Input: part model. Units: mm. Frame: model coordinates. Face numbers are marked on the shaded views. Round coordinates to 2 decimals unless told otherwise and drop trailing zeros. Loops run counter-clockwise (first coordinate to the right, second up) from the corner with the lowest first, then second, coordinate; pieces in that order, holes last.
(1) Line query: line 1 (Y direction, x = 232.1, z = 2.05); line 2 (X direction, y = 23, z = 2.8); line 3 (Z direction, x = 208.5, y = 32). Output: solid intervals per line, ascending.
(2) First-contact query: pin 1 Ø8.5 at (x, y) = (232.1, 71.1) entering from +Z; pin 2 Ø4.5 at (x, y) = (94.1, 23.7) entering from +Z. Flat tips, straight axial feed; report the tip coordinate or a pass-through.
(3) Cut plane C-C, the plane y = 48.5. Output: boundary loops of the cut face in (x, z).
(4) Draft query along Y for the marked faces 1 and 2. Return one class per face: released by +Y, released by -Y, zero draft, split by the parting line, or undercut.
(5) Cut plane A-A, the plane y = 23.7. Output: boundary loops of the cut face in (x, z).
(6) Cut plane B-B, the plane x = 13.6. Output: boundary loops of the cut face in (y, z) (3 decimals).
(7) Cut plane D-D, the plane x = 120. Output: boundary loops of the cut face in (y, z), and give its area (3 significant figures).
from build123d import *

# Parameters (mm, degrees)
SKETCH1_W                = 257.2
SKETCH1_H                = 94.8
BOSS_EXTRUDE1_DEPTH      = 3
SKETCH2_R                = 2.995
BOSS_EXTRUDE2_DEPTH      = 1.4
LPATTERN1_COUNT          = 2
LPATTERN1_PITCH          = 23
LPATTERN1_COUNT_DIR2     = 11
LPATTERN1_PITCH_DIR2     = 23
MIRROR4_COPY_1_SKETCH_R  = 2.995
MIRROR4_COPY_1_DEPTH     = 1.4
MIRROR4_COPY_2_SKETCH_R  = 2.995
MIRROR4_COPY_2_DEPTH     = 1.4
MIRROR4_COPY_3_SKETCH_R  = 2.995
MIRROR4_COPY_3_DEPTH     = 1.4
MIRROR4_COPY_4_SKETCH_R  = 2.995
MIRROR4_COPY_4_DEPTH     = 1.4
MIRROR4_COPY_5_SKETCH_R  = 2.995
MIRROR4_COPY_5_DEPTH     = 1.4
MIRROR4_COPY_6_SKETCH_R  = 2.995
MIRROR4_COPY_6_DEPTH     = 1.4
MIRROR4_COPY_7_SKETCH_R  = 2.995
MIRROR4_COPY_7_DEPTH     = 1.4
MIRROR4_COPY_8_SKETCH_R  = 2.995
MIRROR4_COPY_8_DEPTH     = 1.4
MIRROR4_COPY_9_SKETCH_R  = 2.995
MIRROR4_COPY_9_DEPTH     = 1.4
MIRROR4_COPY_10_SKETCH_R = 2.995
MIRROR4_COPY_10_DEPTH    = 1.4
MIRROR4_COPY_11_SKETCH_R = 2.995
MIRROR4_COPY_11_DEPTH    = 1.4
MIRROR4_COPY_12_SKETCH_R = 2.995
MIRROR4_COPY_12_DEPTH    = 1.4
MIRROR4_COPY_13_SKETCH_R = 2.995
MIRROR4_COPY_13_DEPTH    = 1.4
MIRROR4_COPY_14_SKETCH_R = 2.995
MIRROR4_COPY_14_DEPTH    = 1.4
MIRROR4_COPY_15_SKETCH_R = 2.995
MIRROR4_COPY_15_DEPTH    = 1.4
MIRROR4_COPY_16_SKETCH_R = 2.995
MIRROR4_COPY_16_DEPTH    = 1.4
MIRROR4_COPY_17_SKETCH_R = 2.995
MIRROR4_COPY_17_DEPTH    = 1.4
MIRROR4_COPY_18_SKETCH_R = 2.995
MIRROR4_COPY_18_DEPTH    = 1.4
MIRROR4_COPY_19_SKETCH_R = 2.995
MIRROR4_COPY_19_DEPTH    = 1.4
MIRROR4_COPY_20_SKETCH_R = 2.995
MIRROR4_COPY_20_DEPTH    = 1.4
MIRROR4_COPY_21_SKETCH_R = 2.995
MIRROR4_COPY_21_DEPTH    = 1.4
SKETCH3_R                = 2.7
CUT_EXTRUDE1_DEPTH       = 275.131136502


with BuildPart() as part:
    # Sketch1 → Boss-Extrude1 (new body)
    with BuildSketch(Plane.XY):
        with Locations((128.6, 47.4)):
            Rectangle(SKETCH1_W, SKETCH1_H)
    extrude(amount=BOSS_EXTRUDE1_DEPTH)

    # Sketch2 → Boss-Extrude2 (add)
    with BuildSketch(Plane.XY.offset(3)):
        with Locations((13.6, 12.2)):
            Circle(SKETCH2_R)
    boss_extrude2 = extrude(amount=BOSS_EXTRUDE2_DEPTH)

    # LPattern1: Boss-Extrude2 2 × 11
    with Locations(*[(j * LPATTERN1_PITCH_DIR2, i * LPATTERN1_PITCH, 0) for i in range(LPATTERN1_COUNT) for j in range(LPATTERN1_COUNT_DIR2) if (i, j) != (0, 0)]):
        add(boss_extrude2)

    # Mirror4: Boss-Extrude2 across plane
    add(boss_extrude2.mirror(Plane(origin=(0, 47.4, 0), x_dir=(0, 0, 1), z_dir=(0, -1, 0))))

    # Mirror4 copy 1 sketch → Mirror4 copy 1 (add)
    with BuildSketch(Plane(origin=(23, 94.8, 3), x_dir=(1, 0, 0), z_dir=(0, 0, 1))):
        with Locations((13.6, -12.2)):
            Circle(MIRROR4_COPY_1_SKETCH_R)
    extrude(amount=MIRROR4_COPY_1_DEPTH)

    # Mirror4 copy 2 sketch → Mirror4 copy 2 (add)
    with BuildSketch(Plane(origin=(46, 94.8, 3), x_dir=(1, 0, 0), z_dir=(0, 0, 1))):
        with Locations((13.6, -12.2)):
            Circle(MIRROR4_COPY_2_SKETCH_R)
    extrude(amount=MIRROR4_COPY_2_DEPTH)

    # Mirror4 copy 3 sketch → Mirror4 copy 3 (add)
    with BuildSketch(Plane(origin=(69, 94.8, 3), x_dir=(1, 0, 0), z_dir=(0, 0, 1))):
        with Locations((13.6, -12.2)):
            Circle(MIRROR4_COPY_3_SKETCH_R)
    extrude(amount=MIRROR4_COPY_3_DEPTH)

    # Mirror4 copy 4 sketch → Mirror4 copy 4 (add)
    with BuildSketch(Plane(origin=(92, 94.8, 3), x_dir=(1, 0, 0), z_dir=(0, 0, 1))):
        with Locations((13.6, -12.2)):
            Circle(MIRROR4_COPY_4_SKETCH_R)
    extrude(amount=MIRROR4_COPY_4_DEPTH)

    # Mirror4 copy 5 sketch → Mirror4 copy 5 (add)
    with BuildSketch(Plane(origin=(115, 94.8, 3), x_dir=(1, 0, 0), z_dir=(0, 0, 1))):
        with Locations((13.6, -12.2)):
            Circle(MIRROR4_COPY_5_SKETCH_R)
    extrude(amount=MIRROR4_COPY_5_DEPTH)

    # Mirror4 copy 6 sketch → Mirror4 copy 6 (add)
    with BuildSketch(Plane(origin=(138, 94.8, 3), x_dir=(1, 0, 0), z_dir=(0, 0, 1))):
        with Locations((13.6, -12.2)):
            Circle(MIRROR4_COPY_6_SKETCH_R)
    extrude(amount=MIRROR4_COPY_6_DEPTH)

    # Mirror4 copy 7 sketch → Mirror4 copy 7 (add)
    with BuildSketch(Plane(origin=(161, 94.8, 3), x_dir=(1, 0, 0), z_dir=(0, 0, 1))):
        with Locations((13.6, -12.2)):
            Circle(MIRROR4_COPY_7_SKETCH_R)
    extrude(amount=MIRROR4_COPY_7_DEPTH)

    # Mirror4 copy 8 sketch → Mirror4 copy 8 (add)
    with BuildSketch(Plane(origin=(184, 94.8, 3), x_dir=(1, 0, 0), z_dir=(0, 0, 1))):
        with Locations((13.6, -12.2)):
            Circle(MIRROR4_COPY_8_SKETCH_R)
    extrude(amount=MIRROR4_COPY_8_DEPTH)

    # Mirror4 copy 9 sketch → Mirror4 copy 9 (add)
    with BuildSketch(Plane(origin=(207, 94.8, 3), x_dir=(1, 0, 0), z_dir=(0, 0, 1))):
        with Locations((13.6, -12.2)):
            Circle(MIRROR4_COPY_9_SKETCH_R)
    extrude(amount=MIRROR4_COPY_9_DEPTH)

    # Mirror4 copy 10 sketch → Mirror4 copy 10 (add)
    with BuildSketch(Plane(origin=(230, 94.8, 3), x_dir=(1, 0, 0), z_dir=(0, 0, 1))):
        with Locations((13.6, -12.2)):
            Circle(MIRROR4_COPY_10_SKETCH_R)
    extrude(amount=MIRROR4_COPY_10_DEPTH)

    # Mirror4 copy 11 sketch → Mirror4 copy 11 (add)
    with BuildSketch(Plane(origin=(0, 71.8, 3), x_dir=(1, 0, 0), z_dir=(0, 0, 1))):
        with Locations((13.6, -12.2)):
            Circle(MIRROR4_COPY_11_SKETCH_R)
    extrude(amount=MIRROR4_COPY_11_DEPTH)

    # Mirror4 copy 12 sketch → Mirror4 copy 12 (add)
    with BuildSketch(Plane(origin=(23, 71.8, 3), x_dir=(1, 0, 0), z_dir=(0, 0, 1))):
        with Locations((13.6, -12.2)):
            Circle(MIRROR4_COPY_12_SKETCH_R)
    extrude(amount=MIRROR4_COPY_12_DEPTH)

    # Mirror4 copy 13 sketch → Mirror4 copy 13 (add)
    with BuildSketch(Plane(origin=(46, 71.8, 3), x_dir=(1, 0, 0), z_dir=(0, 0, 1))):
        with Locations((13.6, -12.2)):
            Circle(MIRROR4_COPY_13_SKETCH_R)
    extrude(amount=MIRROR4_COPY_13_DEPTH)

    # Mirror4 copy 14 sketch → Mirror4 copy 14 (add)
    with BuildSketch(Plane(origin=(69, 71.8, 3), x_dir=(1, 0, 0), z_dir=(0, 0, 1))):
        with Locations((13.6, -12.2)):
            Circle(MIRROR4_COPY_14_SKETCH_R)
    extrude(amount=MIRROR4_COPY_14_DEPTH)

    # Mirror4 copy 15 sketch → Mirror4 copy 15 (add)
    with BuildSketch(Plane(origin=(92, 71.8, 3), x_dir=(1, 0, 0), z_dir=(0, 0, 1))):
        with Locations((13.6, -12.2)):
            Circle(MIRROR4_COPY_15_SKETCH_R)
    extrude(amount=MIRROR4_COPY_15_DEPTH)

    # Mirror4 copy 16 sketch → Mirror4 copy 16 (add)
    with BuildSketch(Plane(origin=(115, 71.8, 3), x_dir=(1, 0, 0), z_dir=(0, 0, 1))):
        with Locations((13.6, -12.2)):
            Circle(MIRROR4_COPY_16_SKETCH_R)
    extrude(amount=MIRROR4_COPY_16_DEPTH)

    # Mirror4 copy 17 sketch → Mirror4 copy 17 (add)
    with BuildSketch(Plane(origin=(138, 71.8, 3), x_dir=(1, 0, 0), z_dir=(0, 0, 1))):
        with Locations((13.6, -12.2)):
            Circle(MIRROR4_COPY_17_SKETCH_R)
    extrude(amount=MIRROR4_COPY_17_DEPTH)

    # Mirror4 copy 18 sketch → Mirror4 copy 18 (add)
    with BuildSketch(Plane(origin=(161, 71.8, 3), x_dir=(1, 0, 0), z_dir=(0, 0, 1))):
        with Locations((13.6, -12.2)):
            Circle(MIRROR4_COPY_18_SKETCH_R)
    extrude(amount=MIRROR4_COPY_18_DEPTH)

    # Mirror4 copy 19 sketch → Mirror4 copy 19 (add)
    with BuildSketch(Plane(origin=(184, 71.8, 3), x_dir=(1, 0, 0), z_dir=(0, 0, 1))):
        with Locations((13.6, -12.2)):
            Circle(MIRROR4_COPY_19_SKETCH_R)
    extrude(amount=MIRROR4_COPY_19_DEPTH)

    # Mirror4 copy 20 sketch → Mirror4 copy 20 (add)
    with BuildSketch(Plane(origin=(207, 71.8, 3), x_dir=(1, 0, 0), z_dir=(0, 0, 1))):
        with Locations((13.6, -12.2)):
            Circle(MIRROR4_COPY_20_SKETCH_R)
    extrude(amount=MIRROR4_COPY_20_DEPTH)

    # Mirror4 copy 21 sketch → Mirror4 copy 21 (add)
    with BuildSketch(Plane(origin=(230, 71.8, 3), x_dir=(1, 0, 0), z_dir=(0, 0, 1))):
        with Locations((13.6, -12.2)):
            Circle(MIRROR4_COPY_21_SKETCH_R)
    extrude(amount=MIRROR4_COPY_21_DEPTH)

    # Sketch3 → Cut-Extrude1 (cut, through all)
    with BuildSketch(Plane.XY.offset(3)):
        with Locations((25.1, 71.1)):
            Circle(SKETCH3_R)
        with Locations((94.1, 71.1)):
            Circle(SKETCH3_R)
        with Locations((163.1, 71.1)):
            Circle(SKETCH3_R)
        with Locations((232.1, 71.1)):
            Circle(SKETCH3_R)
    cut_extrude1 = extrude(amount=-CUT_EXTRUDE1_DEPTH, mode=Mode.SUBTRACT)

    # Mirror3: Cut-Extrude1 across plane
    add(cut_extrude1.mirror(Plane(origin=(0, 47.4, 0), x_dir=(0, 0, 1), z_dir=(0, -1, 0))), mode=Mode.SUBTRACT)


solid = part.part
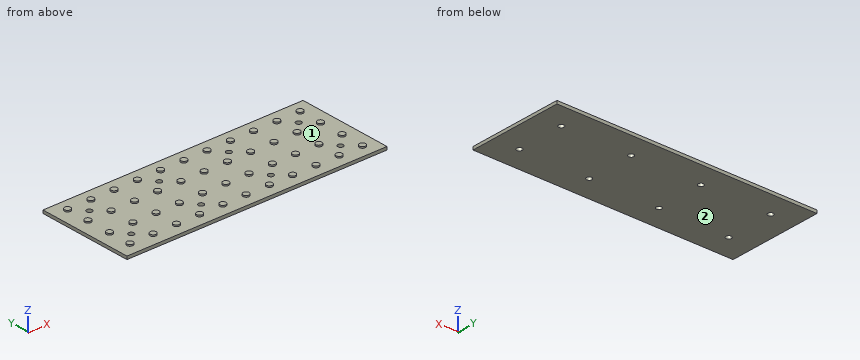
Reported:
1. line 1: y = 0 to 21, 26.4 to 68.4, 73.8 to 94.8
1. line 2: x = 0 to 22.49, 27.71 to 91.49, 96.71 to 160.49, 165.71 to 229.49, 234.71 to 257.2
1. line 3: z = 0 to 3
2. pin 1: stops at z = 3
2. pin 2: passes through
3. outline: (0, 0) - (257.2, 0) - (257.2, 3) - (0, 3) - close
4. face 1: undercut
4. face 2: zero draft
5. outline: (0, 0) - (22.4, 0) - (22.4, 3) - (0, 3) - close; (27.8, 0) - (91.4, 0) - (91.4, 3) - (27.8, 3) - close; (96.8, 0) - (160.4, 0) - (160.4, 3) - (96.8, 3) - close; (165.8, 0) - (229.4, 0) - (229.4, 3) - (165.8, 3) - close; (234.8, 0) - (257.2, 0) - (257.2, 3) - (234.8, 3) - close
6. outline: (0, 0) - (94.8, 0) - (94.8, 3) - (85.595, 3) - (85.595, 4.4) - (79.605, 4.4) - (79.605, 3) - (62.595, 3) - (62.595, 4.4) - (56.605, 4.4) - (56.605, 3) - (38.195, 3) - (38.195, 4.4) - (32.205, 4.4) - (32.205, 3) - (15.195, 3) - (15.195, 4.4) - (9.205, 4.4) - (9.205, 3) - (0, 3) - close
7. outline: (0, 0) - (94.8, 0) - (94.8, 3) - (0, 3) - close
7. area: 284 mm2
